Design review of the part shown in the three views and the two pictorial views. Dimensions are in mm from the part's minimum x, y and z. A direction names the side the tool comes from. Round coordinates to 2 decimals unless told otherwise and drop trailing zeros. Loops run counter-clockwise (first coordinate to the right, second up) from the corner with the lowest first, then second, coordinate; pieces in that order, holes last. Notation, with made-up numbers: (41, 61.25) - (60, 61.25) arc R15 cw to (60, 86.25) - close; hole circle Ø8 at (-24.75, 11.25). An arc over 180 degrees is marked (long way). Return JSON: item names as keys, results as strings. Group by question number.
(1) Wall thickness on L1, parallel to Y at x = 10, z = 4.5; L2, parallel to Z at x = 16.25, y = 11.5; L3, parallel to Y at x = 8.5, z = 1: over which ranges is each line inside the solid? List them lowest first. Write a range as [from, to].
(2) The part is to be moulded in two halves that separate along X. For the marked faces 4, 5 and 6, say which applies: pulls with the +X half, pulls with the -X half, needs draft (parallel to the pull), parting line crosses it, or undercut.
(3) We need section A-A, the plane y = 10. Write out the cut boundary in (x, z), and give its area (3 significant figures).
(4) We need section D-D, the plane z = 3.75. Write out the cut boundary in (x, y), and give its area (3 significant figures).
(5) We need section C-C, the plane z = 17.75. Write out the cut boundary in (x, y).
(6) For the marked faces 1, 2 and 3, list the 3-axis set-ups (+Z, -Z, +X, -X, +Y, -Y) from which the entire face can be reached by the end or side of a thin tool; tool diameter is ignored.
(7) Clearance check with flat-ended pins moving along their axes: pin 1 (6.5 mm diameter, centred on y = 17.5, z = 16.5, fed in from +X); pin 2 (10 mm diameter, centred on y = 7, z = 17, fed in from -X); pin 3 (8 mm diameter, centred on x = 14.5, z = 5, fed in from -Y). State where each tip first meets the part, or that it passes through.
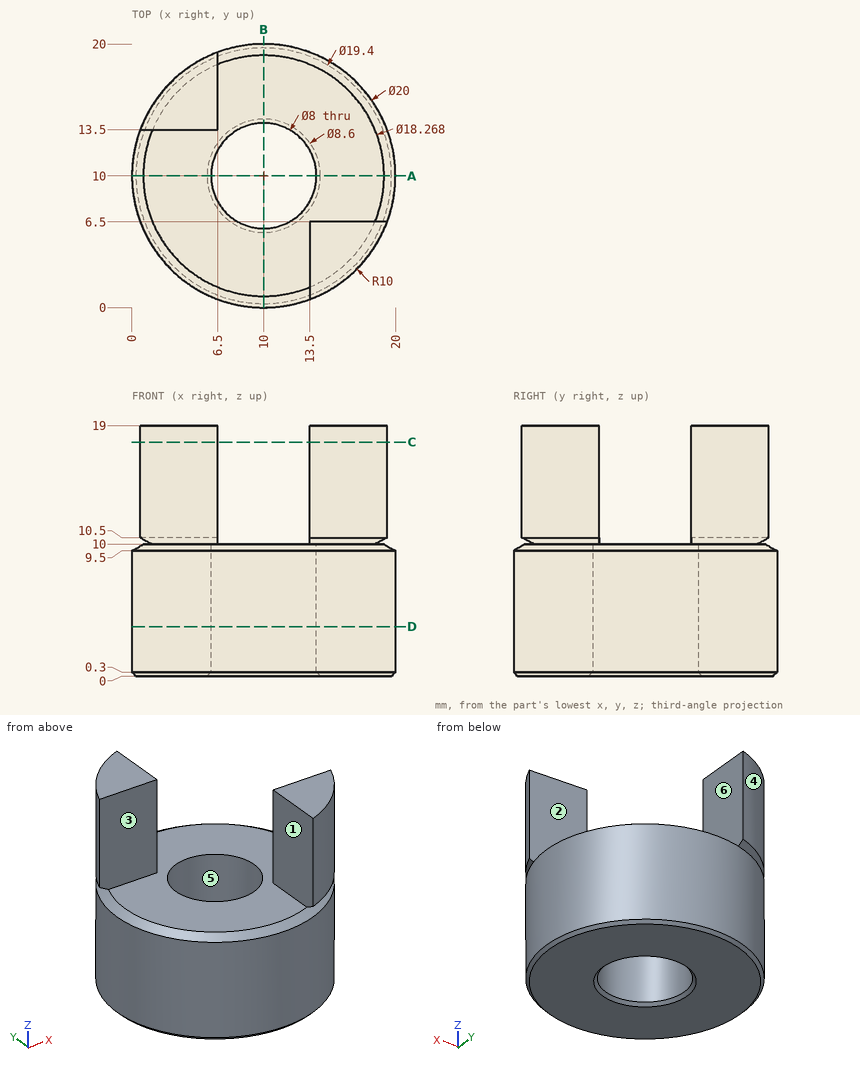
Solutions:
{
 "1": {"L1": "[0, 6], [14, 20]", "L2": "[0, 10]", "L3": "[0.11, 6.29], [13.71, 19.89]"},
 "2": {"face 4": "pulls with the -X half", "face 5": "undercut", "face 6": "pulls with the +X half"},
 "3": {"outline": "(0, 0.3) - (0.3, 0) - (5.7, 0) - (6, 0.3) - (6, 10) - (0.87, 10) - (0, 9.5) - close; (14, 0.3) - (14.3, 0) - (19.7, 0) - (20, 0.3) - (20, 9.5) - (19.13, 10) - (14, 10) - close", "area": "119 mm^2"},
 "4": {"outline": "circle Ø20 at (10, 10); hole circle Ø8 at (10, 10)", "area": "264 mm^2"},
 "5": {"outline": "(0.63, 13.5) - (6.5, 13.5) - (6.5, 19.37) arc R10 ccw to start; (13.5, 0.63) arc R10 ccw to (19.37, 6.5) - (13.5, 6.5) - close"},
 "6": {"face 1": "+Z, -X, +Y, -Y", "face 2": "+Z, +X, -X, +Y", "face 3": "+Z, +X, -X, -Y"},
 "7": {"pin 1": "x = 6.5", "pin 2": "x = 13.5", "pin 3": "y = 0.01"}
}
